Here's the drawing with two shaded views (mm, measured from the low corner). I have some questions. Coordinates: 2 decimals unless noted, no trailing zeros. Write each loop counter-clockwise with the first axis right and the second up, starting at its lowest first coordinate (ties: lowest second). Pieces come first, ordered by that corner, then holes. Notation, with made-up numbers: (-7.75, -28) -> (25.25, -28) arc R22 cw to (25.25, 10) -> close; hole circle Ø5 at (-25, 19.25). An arc over 180 degrees is marked (long way). Put each result on its own line as item: value.
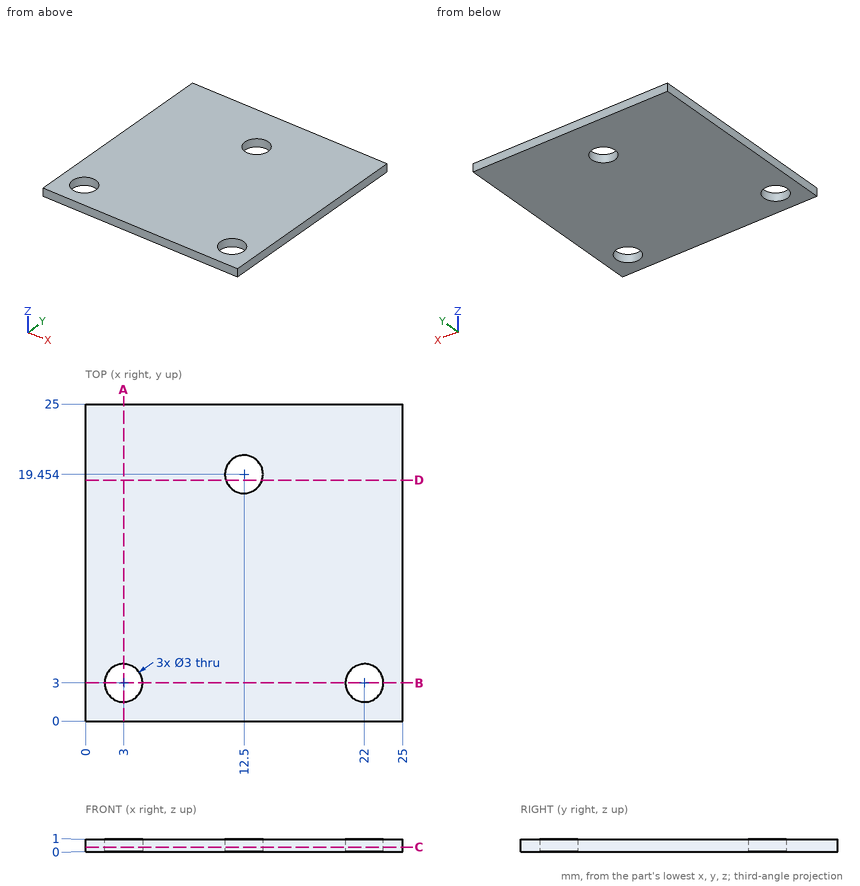
Item 1: Imagine slicing it at C-C on z = 0.35. Write out the boundary of the cut face in (x, y) (1 decimal).
Output:
outline: (0, 0) -> (25, 0) -> (25, 25) -> (0, 25) -> close; hole circle Ø3 at (3, 3); hole circle Ø3 at (12.5, 19.5); hole circle Ø3 at (22, 3)
Item 2: Imagine slicing it at B-B on y = 3. Write out the boundary of the cut face in (x, z), then the cut area to 3 significant figures.
Output:
outline: (0, 0) -> (1.5, 0) -> (1.5, 1) -> (0, 1) -> close; (4.5, 0) -> (20.5, 0) -> (20.5, 1) -> (4.5, 1) -> close; (23.5, 0) -> (25, 0) -> (25, 1) -> (23.5, 1) -> close
area: 19.0 mm²
Item 3: Imagine slicing it at A-A on x = 3. Write out the boundary of the cut face in (y, z), then the cut area to 3 significant figures.
Output:
outline: (0, 0) -> (1.5, 0) -> (1.5, 1) -> (0, 1) -> close; (4.5, 0) -> (25, 0) -> (25, 1) -> (4.5, 1) -> close
area: 22.0 mm²
Item 4: Imagine slicing it at D-D on y = 19. Write out the boundary of the cut face in (x, z).
Output:
outline: (0, 0) -> (11.07, 0) -> (11.07, 1) -> (0, 1) -> close; (13.93, 0) -> (25, 0) -> (25, 1) -> (13.93, 1) -> close
Item 5: Please list where these lines run through material, in increasing order: line 1 along Y through (x, z) = (3, 0.25); line 2 along Y through (x, z) = (12.5, 0.85) (1 decimal); line 3 along X through (y, z) = (18.75, 0.9) (1 decimal). Write a range as from..to.
Output:
line 1: y = 0..1.5, 4.5..25
line 2: y = 0..18, 21..25
line 3: x = 0..11.2, 13.8..25
